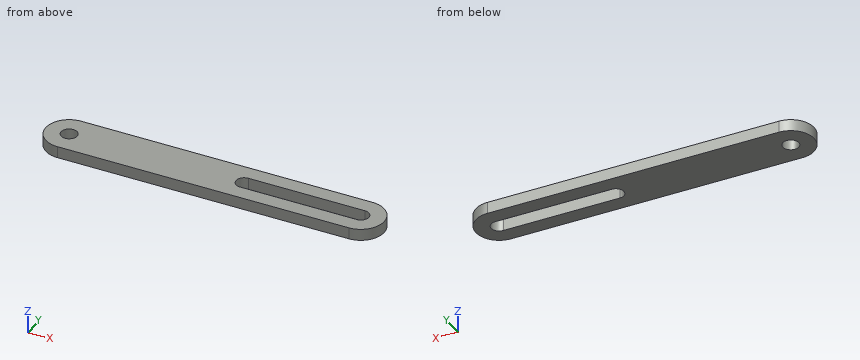
from build123d import *

# Parameters (mm, degrees)
BOSS_EXTRUDE1_DEPTH     = 2.54
CUT_EXTRUDE1_START      = -3.54
SKETCH2_R               = 1.7526
CUT_EXTRUDE1_DEPTH      = 4.54
CUT_EXTRUDE2_DEPTH      = 1
CUT_EXTRUDE2_DEPTH_BACK = 3.54


with BuildPart() as part:
    # Sketch1 → Boss-Extrude1 (new body)
    with BuildSketch(Plane.XY):
        with BuildLine():
            Line((0, 5.08), (63.5, 5.08))
            ThreePointArc((63.5, 5.08), (68.58, 0), (63.5, -5.08))
            Line((63.5, -5.08), (0, -5.08))
            ThreePointArc((0, -5.08), (-5.08, 0), (0, 5.08))
        make_face()
    extrude(amount=BOSS_EXTRUDE1_DEPTH)

    # Sketch2 → Cut-Extrude1 (cut)
    with BuildSketch(Plane.XY.offset(2.54).offset(CUT_EXTRUDE1_START)):
        Circle(SKETCH2_R)
    cut_extrude1 = extrude(amount=CUT_EXTRUDE1_DEPTH, mode=Mode.SUBTRACT)

    # Mirror1: Cut-Extrude1 across plane
    add(cut_extrude1.mirror(Plane(origin=(31.75, 0, 0), x_dir=(0, 0, 1), z_dir=(1, 0, 0))), mode=Mode.SUBTRACT)

    # Sketch4 → Cut-Extrude2 (cut, two sides)
    with BuildSketch(Plane.XY.offset(2.54)) as cut_extrude2_sk:
        with BuildLine():
            Line((63.5, -1.7526), (38.09873006, -1.7526))
            ThreePointArc((38.09873006, -1.7526), (36.34613006, 0), (38.09873006, 1.7526))
            Line((38.09873006, 1.7526), (63.5, 1.7526))
            ThreePointArc((63.5, 1.7526), (65.2526, 0), (63.5, -1.7526))
        make_face()
    extrude(amount=CUT_EXTRUDE2_DEPTH, mode=Mode.SUBTRACT)
    extrude(cut_extrude2_sk.sketch, amount=-CUT_EXTRUDE2_DEPTH_BACK, mode=Mode.SUBTRACT)


solid = part.part
Can you work these out from the model? Positions are in its coordinate system, mm. Give positions to 0.01 mm unless a question says otherwise; leave off trailing zeros. Loops run counter-clockwise (first coordinate to the right, second up) from the corner with the lowest first, then second, coordinate; pieces in that order, holes last. Notation, with made-up numbers: (59.25, 36) -> (100.25, 36) arc R14 cw to (100.25, 43) -> close; hole circle Ø2 at (65.5, 22). An arc over 180 degrees is marked (long way). Return JSON: item names as keys, results as strings.
Q1. I want a section at D-D, the plane y = 4. List the corners of the cut face in (x, z) for me, then the cut area to 3 significant figures.
Checks:
{"outline": "(-3.13, 0) -> (66.63, 0) -> (66.63, 2.54) -> (-3.13, 2.54) -> close", "area": "177 mm2"}
Q2. I want a section at C-C, the plane z = 1.65. List the corners of the cut face in (x, y) for me.
Checks:
{"outline": "(0, -5.08) -> (63.5, -5.08) arc R5.08 ccw to (63.5, 5.08) -> (0, 5.08) arc R5.08 ccw to start; hole circle Ø3.51 at (0, 0); hole (38.1, -1.75) -> (63.5, -1.75) arc R1.75 ccw to (63.5, 1.75) -> (38.1, 1.75) arc R1.75 ccw to start"}
Q3. For pin 1 Ø4 at (x, y) = (5.5, -4) entering from -Z; pin 2 Ø3 at (x, y) = (0, 0) entering from -Z, each with a flat end and sliding along its axis, tell me the tip position at first contact or that it passes through.
Checks:
{"pin 1": "stops at z = 0", "pin 2": "passes through"}
Q4. I want a section at A-A, the plane x = 40. List the corners of the cut face in (y, z) for me.
Checks:
{"outline": "(-5.08, 0) -> (-1.75, 0) -> (-1.75, 2.54) -> (-5.08, 2.54) -> close; (1.75, 0) -> (5.08, 0) -> (5.08, 2.54) -> (1.75, 2.54) -> close"}
Q5. I want a section at B-B, the plane y = 0. List the corners of the cut face in (x, z) for me, then the cut area to 3 significant figures.
Checks:
{"outline": "(-5.08, 0) -> (-1.75, 0) -> (-1.75, 2.54) -> (-5.08, 2.54) -> close; (1.75, 0) -> (36.35, 0) -> (36.35, 2.54) -> (1.75, 2.54) -> close; (65.25, 0) -> (68.58, 0) -> (68.58, 2.54) -> (65.25, 2.54) -> close", "area": "105 mm2"}
Q6. I need wall thicknesses on probe 1 along X at (y, z) = (0, 1.25); probe 2 along Y at (x, z) = (52, 0.1); probe 3 along X at (y, z) = (1.25, 2.3). Which ranges of each line are inside material? Lowest first, please.
Checks:
{"probe 1": "x = -5.08 to -1.75, 1.75 to 36.35, 65.25 to 68.58", "probe 2": "y = -5.08 to -1.75, 1.75 to 5.08", "probe 3": "x = -4.92 to -1.23, 1.23 to 36.87, 64.73 to 68.42"}
